```python
from build123d import *

# Parameters (mm, degrees)
F0_W     = 31.75
F0_H     = 31.75
F1_DEPTH = 25.4
F3_DEPTH = 12.7
F4_W     = 26.9875
F4_H     = 31.75
F5_DEPTH = 6.35
F6_W     = 31.75
F6_H     = 9.525
F7_DEPTH = 25.401
F8_W     = 31.75
F8_H     = 6.35
F9_DEPTH = 25.401


with BuildPart() as f1:
    # F0 (on Top) → F1 (new body)
    with BuildSketch(Plane.XY):
        with Locations((15.875, 15.875)):
            Rectangle(F0_W, F0_H)
    extrude(amount=F1_DEPTH)

    # F2 (on face) → F3 (cut)
    with BuildSketch(Plane.XY.offset(25.4)):
        with BuildLine():
            Line((26.9875, 0), (26.9875, 9.525))
            ThreePointArc((26.9875, 9.525), (15.875, 20.6375), (4.7625, 9.525))
            Line((4.7625, 9.525), (4.7625, 0))
            Line((4.7625, 0), (26.9875, 0))
        make_face()
    extrude(amount=-F3_DEPTH, mode=Mode.SUBTRACT)

    # F4 (on face) → F5 (cut)
    with BuildSketch(Plane.XY.offset(12.7)):
        with Locations((18.25625, 15.875)):
            Rectangle(F4_W, F4_H)
    extrude(amount=F5_DEPTH, mode=Mode.SUBTRACT)

    # F6 (on face) → F7 (cut, through all)
    with BuildSketch(Plane.XY.offset(25.4)):
        with Locations((15.875, 4.7625)):
            Rectangle(F6_W, F6_H)
    extrude(amount=-F7_DEPTH, mode=Mode.SUBTRACT)

    # F8 (on Top) → F9 (cut, through all)
    with BuildSketch(Plane.XY):
        with Locations((15.875, 28.575)):
            Rectangle(F8_W, F8_H)
    extrude(amount=F9_DEPTH, mode=Mode.SUBTRACT)


solid = f1.part
```
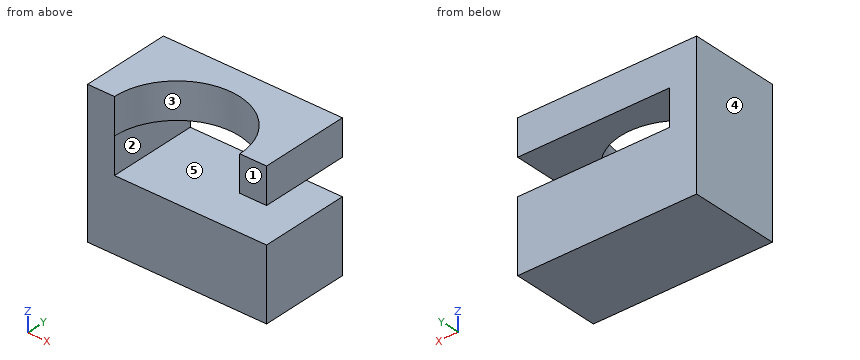
Build history of the part. All positions in model axes, mm. Face numbers are marked on the shaded views. A direction names the side the tool comes from. Round coordinates to 2 decimals unless told otherwise and drop trailing zeros. Write each loop counter-clockwise with the first axis right and the second up, starting at its lowest first coordinate (ties: lowest second). Pieces come first, ordered by that corner, then holes.
1) 3-axis set-ups, long thin cutter, end or side, ignore diameter. For the marked faces 1 and 2: which of +Z, -Z, +X, -X, +Y, -Y reach the whole face in a straight line?
2) Drill centre lines: probe 1 along Z at (x, y) = (26.5, 20.5); probe 2 along Z at (x, y) = (6, 11.5); probe 3 along X at (y, z) = (14, 18). Where is each one in solid material? Low to high.
3) Band-saw the part on B-B, the plane y = 16. List the corners of the cut face in (x, z), and give its area (3 significant figures).
4) Band-saw the part on D-D, the plane y = 23.5. List the corners of the cut face in (x, z), and give its area (3 significant figures).
5) Mould opens along X. For the marked faces 3, 4 and 5 say: +X half, -X half, draft (parallel to the pull), parting line (faces both ways), or undercut.
6) Pin check, flat tips, straight feed: pin 1 (8 mm diameter, centred on x = 20.5, z = 15, fed in from +Y); pin 2 (3 mm diameter, centred on x = 17.5, z = 18.5, fed in from -Y). Stop position of each tip, or through.
7) Band-saw the part on A-A, the plane x = 28. List the corners of the cut face in (y, z) (3 decimals), and give its area (3 significant figures).
Ans:
1. face 1: +Z, -Z, +X, -X, -Y
1. face 2: +X, +Y, -Y
2. probe 1: z = 0 to 12.7, 19.05 to 25.4
2. probe 2: z = 0 to 12.7
2. probe 3: x = 0 to 4.76
3. outline: (0, 0) - (31.75, 0) - (31.75, 12.7) - (4.76, 12.7) - (4.76, 19.05) - (6.84, 19.05) - (6.84, 25.4) - (0, 25.4) - close; (24.91, 19.05) - (31.75, 19.05) - (31.75, 25.4) - (24.91, 25.4) - close
3. area: 520 mm2
4. outline: (0, 0) - (31.75, 0) - (31.75, 12.7) - (4.76, 12.7) - (4.76, 19.05) - (31.75, 19.05) - (31.75, 25.4) - (0, 25.4) - close
4. area: 635 mm2
5. face 3: undercut
5. face 4: -X half
5. face 5: draft
6. pin 1: stops at y = 25.4
6. pin 2: stops at y = 20.22
7. outline: (9.525, 0) - (25.4, 0) - (25.4, 12.7) - (9.525, 12.7) - close; (9.525, 19.05) - (25.4, 19.05) - (25.4, 25.4) - (9.525, 25.4) - close
7. area: 302 mm2
